Source: CAD feature listing. Evaluate the final solid. Frame: model axes, mm. A direction names the side the tool comes from. Give positions to 0.01 mm unless a question says otherwise; leave off trailing zeros. Order: outer loops, then holes, each group sorted by start corner. A loop starts at its lowest first (then second) coordinate and runs counter-clockwise, first axis right, second up.
1) First-contact query: P1, Ø1, axis at y = 11, z = 31.5, coming from the +X side; P2, Ø3, axis at y = 40, z = 15, coming from the -X side; P3, Ø8, axis at y = 18.5, z = 36.5, coming from the +X side. Flat tips, straight axial feed; report the tip coordinate or a pass-through.
2) Section D-D, the plane z = -19. Return loops of the section in (x, y), plus the area to 3 significant figures.
3) Access query for faces 1 (the face through (50, 3.81, 0)), 2 (the face through (36, 0, 0)), 3 (the face through (55, 26, -12.7)), 4 (the face through (44.797, 26.332, -0.876)). Directions: +Z, -Z, +X, -X, +Y, -Y. A direction counts if a zero-diameter tool reaches every point of the face in a straight line with its end or side. Return the directions, or none.
4) Draft query along Z for faces 5 (the face through (55, 26, 12.7)), 6 (the face through (50.497, 25.098, 0.196)), 7 (the face through (38.6, 26.3, -0.8)), 8 (the face through (38.4, 2.54, -6.3)). Return one class per face: released by +Z, released by -Z, zero draft, split by the parting line, or undercut.
5) Material intervals for line 1 (X direction, y = 20, z = 2); line 2 (Z direction, x = 28.5, y = 8); line 3 (Z direction, x = 31.5, y = 22.5), sorted ascending.
6) Section C-C, the plane z = 11. Return loops of the section in (x, y), plus the area to 3 significant figures.
7) Section B-B, the plane y = 20.5. Return loops of the section in (x, z), plus the area to 3 significant figures.
8) Section A-A, the plane x = 22.5. Return loops of the section in (y, z), plus the area to 3 significant figures.
Autodesk Inventor part; units mm, degrees
ref_plane "YZ Plane" through (0, 0, 0) normal (1, 0, 0) x (0, 1, 0)
ref_plane "XZ Plane" through (0, 0, 0) normal (0, 1, 0) x (-1, 0, 0)
ref_plane "XY Plane" through (0, 0, 0) normal (0, 0, 1) x (1, 0, 0)
sketch "Sketch1" plane through (0, 0, 0) normal (0, 1, 0) x (-1, 0, 0)
  arc A0 (-8.442, 47.877) -> (-8.442, -47.877) centre (0, 0) ccw
  arc A1 (-7.7804, 44.1249) -> (-7.7804, -44.1249) centre (0, 0) ccw
  arc A2 (-6.7042, 38.0215) -> (-6.7042, -38.0215) centre (0, 0) ccw
  arc A3 (-6.0426, 34.2693) -> (-6.0426, -34.2693) centre (0, 0) ccw
  line L0 (0, 0) -> (57.6746, 0) construction
  line L1 (-10.0151, -56.7984) -> (0, 0)
  line L2 (0, 0) -> (-10.8029, 61.2664)
  line L3 (0, 0) -> (62.2115, 0) construction
  dimension "d0" = 97.2312
  dimension "d1" = 89.6112
  dimension "d14" = 77.216
  dimension "d15" = 69.596
  dimension "d17" = 100
  dimension "d18" = 100
extrude "Extrusion1" add sketch "Sketch1" along normal blind 50.8 contours L2 A1 L1 A0 | L2 A3 L1 A2
sketch "Sketch2" plane through (0, 0, 0) normal (0, 0, 1) x (1, 0, 0)
  line L0 (0, 0) -> (58.8549, 0)
  line L1 (58.8549, 0) -> (58.8549, 25.4)
  line L2 (0, 25.4) -> (0, 0)
  line L3 (50.4953, 3.81) -> (3.81, 3.81)
  line L4 (3.81, 3.81) -> (3.81, 21.59)
  line L5 (3.81, 21.59) -> (45.975, 21.59)
  line L6 (45.975, 21.59) -> (45.975, 3.81)
  line L7 (45.975, 21.59) -> (45.975, 25.4)
  line L8 (45.975, 3.81) -> (45.975, 0)
  line L9 (50.4953, 21.59) -> (50.4953, 3.81)
  line L10 (0, 50.8) -> (58.8549, 50.8)
  line L11 (58.8549, 50.8) -> (58.8549, 25.4)
  line L12 (50.4953, 46.99) -> (3.81, 46.99)
  line L13 (3.81, 29.21) -> (45.975, 29.21)
  line L14 (45.975, 29.21) -> (45.975, 46.99)
  line L15 (45.975, 29.21) -> (45.975, 25.4)
  line L16 (45.975, 46.99) -> (45.975, 50.8)
  line L17 (50.4953, 29.21) -> (50.4953, 46.99)
  line L18 (50.4953, 29.21) -> (50.4953, 21.59)
  line L19 (45.975, 25.4) -> (0, 25.4)
extrude "Extrusion2" add sketch "Sketch2" along normal mid plane 25.4 contours L8 L3 L9 L18 L17 L12 L16 L10 L11 L1 L0
sketch "Sketch3" plane through (0, 0, 0) normal (0, -1, 0) x (1, 0, 0)
  circle A0 centre (0, 0) radius 44.8056
  circle A1 centre (0, 0) radius 38.608
  line L0 (7.7804, -44.1249) -> (6.0426, -34.2693)
  line L1 (6.0426, 34.2693) -> (6.7042, 38.0215)
  line L2 (6.7042, 38.0215) -> (7.7804, 44.1249)
  point P0 (6.7042, -38.0215)
  dimension "d7" = 77.216
extrude "Extrusion3" add sketch "Sketch3" against normal blind 2.54 contours A0 L0 A1 L2 picked at (42.4436, 2.9594)
sketch "Sketch4" plane through (0, 50.8, 0) normal (0, 1, 0) x (1, 0, 0)
  line L0 (58.8549, -12.7) -> (58.8549, 12.7)
  arc A0 (58.8549, 12.7) -> (58.8549, -12.7) centre (76.984, 0) ccw
  point P0 (0, 0)
sketch "Sketch5" plane through (46.9275, 3.81, 12.7) normal (0, 1, 0) x (1, 0, 0)
  arc A0 (6.5029, 25.4) -> (6.6061, 0) centre (32.0653, 12.8036) ccw
  line L0 (6.5029, 25.4) -> (1.7839, 25.4)
  line L1 (0, 25.4) -> (3.5678, 25.4)
  line L2 (1.7839, 25.4) -> (2.3688, 0)
  line L3 (3.5678, 0) -> (0, 0)
  line L4 (6.6061, 0) -> (2.3688, 0)
  point P0 (-46.9275, 12.7)
  point P1 (6.5578, 0.0965)
extrude "Extrusion4" cut sketch "Sketch5" along normal up to surface (43.18 mm away)
extrude "Extrusion5" cut sketch "Sketch4" against normal up to surface (50.8 mm away)
properties part number "Mount"
From the geometry:
1. P1: stops at x = 37.45
1. P2: stops at x = 30.64
1. P3: stops at x = 36.16
2. outline: (29.15, 0) - (44.75, 0) - (44.75, 50.8) - (40.58, 50.8) - (40.58, 2.54) - (33.61, 2.54) - (33.61, 50.8) - (29.15, 50.8) - close
2. area: 456 mm2
3. face 1: none
3. face 2: +Z, -Z, +X, -X, -Y
3. face 3: -Z, +X, +Y, -Y
3. face 4: +Y
4. face 5: released by +Z
4. face 6: split by the parting line
4. face 7: undercut
4. face 8: undercut
5. line 1: x = 34.74 to 38.56, 44.76 to 48.57, 50.57 to 54.94
5. line 2: z = -39.39 to -34.57, -26.04 to -19.97, 19.97 to 26.04, 34.57 to 39.39
5. line 3: z = -37.03 to -31.86, -22.32 to -14.79, 14.79 to 22.32, 31.86 to 37.03
6. outline: (33.01, 0) - (57.78, 0) - (57.78, 50.8) - (43.43, 50.8) - (43.43, 2.54) - (37.01, 2.54) - (37.01, 50.8) - (33.01, 50.8) - close; hole (47.35, 3.81) - (52.75, 3.81) - (52.75, 46.99) - (47.35, 46.99) - close
6. area: 715 mm2
7. outline: (6.04, -34.27) - (6.7, -38.02) arc R38.61 ccw to (6.7, 38.02) - (6.04, 34.27) arc R34.8 cw to start; (7.78, -44.12) - (8.44, -47.88) arc R48.62 ccw to (8.44, 47.88) - (7.78, 44.12) arc R44.81 cw to start; (53.43, -12.7) - (58.85, -12.7) arc R22.13 cw to (58.85, 12.7) - (53.53, 12.7) arc R28.5 ccw to start
7. area: 1,010 mm2
8. outline: (0, -43.1) - (50.8, -43.1) - (50.8, -38.75) - (2.54, -38.75) - (2.54, -31.37) - (50.8, -31.37) - (50.8, -26.55) - (0, -26.55) - close; (0, 26.55) - (50.8, 26.55) - (50.8, 31.37) - (2.54, 31.37) - (2.54, 38.75) - (50.8, 38.75) - (50.8, 43.1) - (0, 43.1) - close
8. area: 970 mm2
